```python
from build123d import *

# Parameters (mm, degrees)
SKETCH_1_W             = 215
SKETCH_1_H             = 10
SM_BASE_FLANGE_1_DEPTH = 2
SKETCH_6_R             = 2.5
CUT_EXTRUDE_1_DEPTH    = 108.634799205
FILLET_1_R             = 5


# Sheet-metal steps are written as plain solids
with BuildPart() as part:
    # Sketch 1 → Базовая кромка1 (new body)
    with BuildSketch(Plane.XY):
        Rectangle(SKETCH_1_W, SKETCH_1_H)
    extrude(amount=-SM_BASE_FLANGE_1_DEPTH)

    # Эскиз6 → Вырез-Вытянуть1 (cut, through all)
    with BuildSketch(Plane.XY):
        with Locations((100, 0)):
            Circle(SKETCH_6_R)
        with Locations(Location((-100, 0, 0), (0, 0, 180))):
            Circle(SKETCH_6_R)
    extrude(amount=-CUT_EXTRUDE_1_DEPTH, mode=Mode.SUBTRACT)

    # Скругление1
    fillet_1_edges = [part.edges().sort_by_distance(p)[0] for p in [
        (107.5, -5, -1),
        (107.5, 5, -1),
        (-107.5, -5, -1),
        (-107.5, 5, -1),
    ]]
    fillet(fillet_1_edges, radius=FILLET_1_R - 0.0001)  # a hair under: the kernel refuses the full size


solid = part.part
```
Part model, mm, in its own coordinate system. Round coordinates to 2 decimals unless told otherwise and drop trailing zeros. Loops run counter-clockwise (first coordinate to the right, second up) from the corner with the lowest first, then second, coordinate; pieces in that order, holes last. Notation, with made-up numbers: (54, -0.75) -> (80, -0.75) arc R18 ccw to (80, 21.25) -> close; hole circle Ø4 at (86.25, -22). An arc over 180 degrees is marked (long way). Use CSV: the item, a comma, the result in double quotes. Start each with the question number.
1) Wall check: L1, parallel to Y at x = 100, z = -1.15; L2, parallel to X at y = -2, z = -1; L3, parallel to X at y = 0.5, z = -1.65. Give the ranges that are in metal, low to high. Write a range as [from, to].
2) Pull direction X, two halves, no side cores. Call faces 1 (the cylindrical face through (106, -3.57, -1.01)), 2 (the cylindrical face through (102.385, 0.751, -0.986)), 3 (the cylindrical face through (-106.07, -3.5, -1.01)): +X half, -X half, draft (parallel to the pull), parting line (faces both ways), or undercut.
3) Drop a flat-ended pin along its axis: P1, Ø4.5, axis at x = 100, y = 0, coming from the +Z side. Give the stop position or say it passes through.
4) Cut at B-B, the plane x = 100. Write the cut outline in (y, z), plus the area to 3 significant figures.
5) Cut at A-A, the plane z = -1.4. Give the number of separate pieces and of enclosed holes in the cut face, plus the area to 3 significant figures.
Determined:
1,L1,"y = [-5, -2.5], [2.5, 5]"
1,L2,"x = [-107.08, -101.5], [-98.5, 98.5], [101.5, 107.08]"
1,L3,"x = [-107.47, -102.45], [-97.55, 97.55], [102.45, 107.47]"
2,face 1,"+X half"
2,face 2,"undercut"
2,face 3,"-X half"
3,P1,"passes through"
4,outline,"(-5, -2) -> (-2.5, -2) -> (-2.5, 0) -> (-5, 0) -> close; (2.5, -2) -> (5, -2) -> (5, 0) -> (2.5, 0) -> close"
4,area,"10.0 mm2"
5,separate pieces,"1"
5,enclosed holes,"2"
5,area,"2,090 mm2"
